```python
from build123d import *

# Parameters (mm, degrees)
SKETCH1_W           = 215
SKETCH1_H           = 115
BOSS_EXTRUDE1_DEPTH = 49
SKETCH2_R           = 16.899563319
CUT_EXTRUDE1_DEPTH  = 1
SKETCH4_W           = 15
SKETCH4_H           = 111
CUT_EXTRUDE2_DEPTH  = 40


with BuildPart() as part:
    # Sketch1 → Boss-Extrude1 (new body)
    with BuildSketch(Plane(origin=(0, 0, 0), x_dir=(1, 0, 0), z_dir=(0, 1, 0))):
        Rectangle(SKETCH1_W, SKETCH1_H)
    extrude(amount=BOSS_EXTRUDE1_DEPTH)

    # Sketch2 → Cut-Extrude1 (cut)
    with BuildSketch(Plane(origin=(0, 49, 0), x_dir=(1, 0, 0), z_dir=(0, 1, 0))):
        with Locations(Location((-73.794759825, -26.100436681, 0), (0, 0, 270))):
            Circle(SKETCH2_R)
    extrude(amount=-CUT_EXTRUDE1_DEPTH, mode=Mode.SUBTRACT)

    # Sketch4 → Cut-Extrude2 (cut)
    with BuildSketch(Plane(origin=(0, 49, 0), x_dir=(1, 0, 0), z_dir=(0, 1, 0))):
        with Locations((100, 0)):
            Rectangle(SKETCH4_W, SKETCH4_H)
    extrude(amount=-CUT_EXTRUDE2_DEPTH, mode=Mode.SUBTRACT)


solid = part.part
```
Can you work these out from the model? Positions are in its coordinate system, mm. A direction names the side the tool comes from. Coordinates: 2 decimals unless noted, no trailing zeros. Loops run counter-clockwise (first coordinate to the right, second up) from the corner with the lowest first, then second, coordinate; pieces in that order, holes last. Notation, with made-up numbers: (26.5, -5) - (32.5, -5) arc R24 cw to (32.5, 14) - close; hole circle Ø2 at (-22.75, -26). An arc over 180 degrees is marked (long way). Use a Markdown table: item, result.
Item 1: If I drill on probe 1 along X at (y, z) = (10.5, -53); probe 2 along Y at (x, z) = (-88, 34), over which ranges is the centre line in solid material (lowest first)? Write a range as from..to.
Numbers:
| item | result |
|---|---|
| probe 1 | x = -107.5..92.5 |
| probe 2 | y = 0..48 |
Item 2: Will these pins go through, and if not, where does the flat tip stop? pin 1 (7.5 mm diameter, centred on x = 101.5, z = -22, fed in from +Y); pin 2 (2 mm diameter, centred on x = 65, z = 10.5, fed in from -Y); pin 3 (6 mm diameter, centred on y = 20, z = -44.5, fed in from +X).
Numbers:
| item | result |
|---|---|
| pin 1 | stops at y = 9 |
| pin 2 | stops at y = 0 |
| pin 3 | stops at x = 92.5 |
Item 3: I want a section at C-C on z = 38. Please give me the cut outline in (x, y).
Numbers:
| item | result |
|---|---|
| outline | (-107.5, 0) - (107.5, 0) - (107.5, 9) - (92.5, 9) - (92.5, 49) - (-61.79, 49) - (-61.79, 48) - (-85.79, 48) - (-85.79, 49) - (-107.5, 49) - close |
Item 4: I want a section at A-A on y = 46. Please give me the cut outline in (x, z).
Numbers:
| item | result |
|---|---|
| outline | (-107.5, -57.5) - (107.5, -57.5) - (107.5, -55.5) - (92.5, -55.5) - (92.5, 55.5) - (107.5, 55.5) - (107.5, 57.5) - (-107.5, 57.5) - close |
Item 5: I want a section at D-D on z = 14. Please give me the cut outline in (x, y).
Numbers:
| item | result |
|---|---|
| outline | (-107.5, 0) - (107.5, 0) - (107.5, 9) - (92.5, 9) - (92.5, 49) - (-62, 49) - (-62, 48) - (-85.59, 48) - (-85.59, 49) - (-107.5, 49) - close |
Item 6: We'd pull the mould along X, two halves only. Please class faces 1 (the face through (-107.5, 24, 1)), 2 (the face through (-74, 48, 26)), 3 (the face through (-2, 24, 57.5)): released by +X, released by -X, zero draft, split by the parting line, or undercut.
Numbers:
| item | result |
|---|---|
| face 1 | released by -X |
| face 2 | undercut |
| face 3 | zero draft |
Item 7: I want a section at B-B on z = -13. Please give me the cut outline in (x, y), and give its area (4 significant figures).
Numbers:
| item | result |
|---|---|
| outline | (-107.5, 0) - (107.5, 0) - (107.5, 9) - (92.5, 9) - (92.5, 49) - (-107.5, 49) - close |
| area | 9,935 mm2 |
Item 8: For faces 4 (the face through (-2, 0, -1)), 5 (the face through (100, 29, -55.5)), 6 (the face through (-59.545, 48.507, 35.186)), which set-ups out of +Z, -Z, +X, -X, +Y, -Y let a thin tool reach every point of the face, with its end or its side?
Numbers:
| item | result |
|---|---|
| face 4 | +Z, -Z, +X, -X, -Y |
| face 5 | +X, +Y |
| face 6 | +Y |
